Geometry check sheet. Reference: the model listing, model coordinates, mm. Face numbers are marked on the shaded views. A direction names the side the tool comes from. Give positions to 0.01 mm unless a question says otherwise; leave off trailing zeros. Write each loop counter-clockwise with the first axis right and the second up, starting at its lowest first coordinate (ties: lowest second). Pieces come first, ordered by that corner, then holes. Notation, with made-up numbers: (34, 12.25) -> (74, 12.25) arc R26 ccw to (74, 37.25) -> close; hole circle Ø7 at (66, 27.25). An arc over 180 degrees is marked (long way). One line per item, written item: value.
from build123d import *

# Parameters (mm, degrees)
SKETCH1_W           = 21
SKETCH1_H           = 16
SKETCH1_W_2         = 17
SKETCH1_H_2         = 12
BOSS_EXTRUDE1_DEPTH = 2
SKETCH1_6_W         = 21
SKETCH1_6_H         = 16
SKETCH1_6_W_2       = 17
SKETCH1_6_H_2       = 12
BOSS_EXTRUDE2_DEPTH = 7
SKETCH2_W           = 41
SKETCH2_H           = 16
BOSS_EXTRUDE3_DEPTH = 2
SKETCH3_W           = 3.5
SKETCH3_H           = 2
CUT_EXTRUDE1_DEPTH  = 33.954514107
SKETCH4_W           = 3.5
SKETCH4_H           = 8
CUT_EXTRUDE2_DEPTH  = 1
CUT_EXTRUDE3_START  = -7
SKETCH5_W           = 2
SKETCH5_H           = 8
SKETCH5_H_2         = 6
CUT_EXTRUDE3_DEPTH  = 7
CUT_EXTRUDE4_DEPTH  = 2
CUT_EXTRUDE5_DEPTH  = 2
SKETCH9_W           = 4
SKETCH9_H           = 4
BOSS_EXTRUDE4_DEPTH = 7
SKETCH10_R          = 0.5
CUT_EXTRUDE6_DEPTH  = 35.84250278
SKETCH11_W          = 3.5
SKETCH11_H          = 8
CUT_EXTRUDE7_DEPTH  = 1
FILLET1_R           = 2


with BuildPart() as part:
    # Sketch1 → Boss-Extrude1 (new body)
    # profile 1 of 2: a face of its own
    with BuildSketch(Plane(origin=(0, 0, 0), x_dir=(1, 0, 0), z_dir=(0, 1, 0))):
        with Locations((-8.5, 6)):
            Rectangle(SKETCH1_W, SKETCH1_H)
        with Locations((-8.5, 6)):
            Rectangle(SKETCH1_W_2, SKETCH1_H_2, mode=Mode.SUBTRACT)
    # profile 2 of 2: a face of its own
    with BuildSketch(Plane(origin=(0, 0, 0), x_dir=(1, 0, 0), z_dir=(0, 1, 0))):
        with Locations((-8.5, 6)):
            Rectangle(SKETCH1_W_2, SKETCH1_H_2)
    extrude(amount=BOSS_EXTRUDE1_DEPTH)

    # Sketch1<6> → Boss-Extrude2 (add)
    with BuildSketch(Plane(origin=(0, 0, 0), x_dir=(1, 0, 0), z_dir=(0, 1, 0))):
        with Locations((-8.5, 6)):
            Rectangle(SKETCH1_6_W, SKETCH1_6_H)
        with Locations((-8.5, 6)):
            Rectangle(SKETCH1_6_W_2, SKETCH1_6_H_2, mode=Mode.SUBTRACT)
    extrude(amount=BOSS_EXTRUDE2_DEPTH)

    # Sketch2 → Boss-Extrude3 (add)
    with BuildSketch(Plane.XZ):
        with Locations((-8.5, -6)):
            Rectangle(SKETCH2_W, SKETCH2_H)
    extrude(amount=BOSS_EXTRUDE3_DEPTH)

    # Sketch3 → Cut-Extrude1 (cut, through all)
    with BuildSketch(Plane(origin=(0, 0, 0), x_dir=(1, 0, 0), z_dir=(0, 1, 0))):
        with Locations((-24.75, 11)):
            Rectangle(SKETCH3_W, SKETCH3_H)
        with Locations((-24.75, 1)):
            Rectangle(SKETCH3_W, SKETCH3_H)
        with Locations((7.75, 11)):
            Rectangle(SKETCH3_W, SKETCH3_H)
        with Locations((7.75, 1)):
            Rectangle(SKETCH3_W, SKETCH3_H)
    extrude(amount=-CUT_EXTRUDE1_DEPTH, mode=Mode.SUBTRACT)

    # Sketch4 → Cut-Extrude2 (cut)
    with BuildSketch(Plane.XZ.offset(2)):
        with Locations((-24.75, -6)):
            Rectangle(SKETCH4_W, SKETCH4_H)
    extrude(amount=-CUT_EXTRUDE2_DEPTH, mode=Mode.SUBTRACT)

    # Sketch5 → Cut-Extrude3 (cut)
    with BuildSketch(Plane(origin=(0, 7, 0), x_dir=(1, 0, 0), z_dir=(0, 1, 0)).offset(CUT_EXTRUDE3_START)):
        with Locations((-18, 6)):
            Rectangle(SKETCH5_W, SKETCH5_H)
        with Locations((1, 9)):
            Rectangle(SKETCH5_W, SKETCH5_H_2)
    extrude(amount=CUT_EXTRUDE3_DEPTH, mode=Mode.SUBTRACT)

    # Sketch7 → Cut-Extrude4 (cut)
    with BuildSketch(Plane(origin=(0, 2, 0), x_dir=(1, 0, 0), z_dir=(0, 1, 0))):
        Polygon((-17, 2), (-17, 0), (0, 0), (0, 6), (0, 12), (-17, 12), (-17, 10), align=None)
    extrude(amount=-CUT_EXTRUDE4_DEPTH, mode=Mode.SUBTRACT)

    # Sketch8 → Cut-Extrude5 (cut)
    with BuildSketch(Plane(origin=(0, 7, 0), x_dir=(1, 0, 0), z_dir=(0, 1, 0))):
        Polygon((-17, 2), (-19, 2), (-19, -2), (2, -2), (2, 6), (0, 6), (0, 0), (-17, 0), align=None)
        Polygon((-19, 10), (-17, 10), (-17, 12), (2, 12), (2, 14), (-19, 14), align=None)
    extrude(amount=-CUT_EXTRUDE5_DEPTH, mode=Mode.SUBTRACT)

    # Sketch9 → Boss-Extrude4 (add)
    with BuildSketch(Plane(origin=(0, 5, 0), x_dir=(1, 0, 0), z_dir=(0, 1, 0))):
        with Locations((-17, 16)):
            Rectangle(SKETCH9_W, SKETCH9_H)
        with Locations((0, 16)):
            Rectangle(SKETCH9_W, SKETCH9_H)
        with Locations((0, -4)):
            Rectangle(SKETCH9_W, SKETCH9_H)
        with Locations((-17, -4)):
            Rectangle(SKETCH9_W, SKETCH9_H)
    extrude(amount=-BOSS_EXTRUDE4_DEPTH)

    # Sketch10 → Cut-Extrude6 (cut, through all)
    with BuildSketch(Plane(origin=(0, 5, 0), x_dir=(1, 0, 0), z_dir=(0, 1, 0))):
        with Locations(Location((-17, 16, 0), (0, 0, 270))):
            Circle(SKETCH10_R)
        with Locations(Location((0, 16, 0), (0, 0, 270))):
            Circle(SKETCH10_R)
        with Locations(Location((0, -4, 0), (0, 0, 270))):
            Circle(SKETCH10_R)
        with Locations(Location((-17, -4, 0), (0, 0, 270))):
            Circle(SKETCH10_R)
    extrude(amount=-CUT_EXTRUDE6_DEPTH, mode=Mode.SUBTRACT)

    # Sketch11 → Cut-Extrude7 (cut)
    with BuildSketch(Plane.XZ.offset(2)):
        with Locations((7.75, -6)):
            Rectangle(SKETCH11_W, SKETCH11_H)
    extrude(amount=-CUT_EXTRUDE7_DEPTH, mode=Mode.SUBTRACT)

    # Fillet1
    fillet1_edges = [part.edges().sort_by_distance(p)[0] for p in [
        (-29, -1, 2),
        (-29, -1, -14),
        (12, -1, -14),
        (12, -1, 2),
    ]]
    fillet(fillet1_edges, radius=FILLET1_R)


solid = part.part
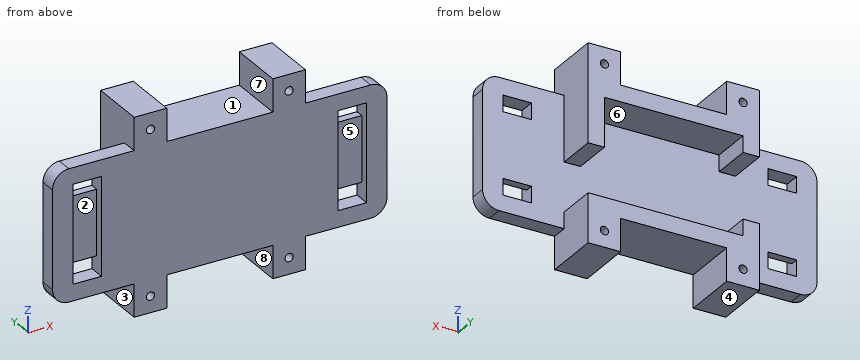
1) Sectioned sample at C-C on z = -16. Record the cut outline in (x, y).
Verdict:
outline: (-19, -2) -> (-17.5, -2) -> (-17.5, 5) -> (-19, 5) -> close; (-16.5, -2) -> (-15, -2) -> (-15, 5) -> (-16.5, 5) -> close; (-2, -2) -> (-0.5, -2) -> (-0.5, 5) -> (-2, 5) -> close; (0.5, -2) -> (2, -2) -> (2, 5) -> (0.5, 5) -> close
2) Sectioned sample at A-A on y = 1.5. Record the cut outline in (x, z).
Verdict:
outline: (-19, -18) -> (-15, -18) -> (-15, -14) -> (-2, -14) -> (-2, -18) -> (2, -18) -> (2, -12) -> (-17, -12) -> (-17, -10) -> (-19, -10) -> close; (-19, -2) -> (-17, -2) -> (-17, 0) -> (0, 0) -> (0, -6) -> (2, -6) -> (2, 6) -> (-2, 6) -> (-2, 2) -> (-15, 2) -> (-15, 6) -> (-19, 6) -> close; hole circle Ø1 at (-17, -16); hole circle Ø1 at (-17, 4); hole circle Ø1 at (0, -16); hole circle Ø1 at (0, 4)
3) Sectioned sample at B-B on z = -5.25. Record the cut outline in (x, y), plus the area to 3 significant figures.
Verdict:
outline: (-29, -2) -> (-26.5, -2) -> (-26.5, -1) -> (-23, -1) -> (-23, -2) -> (6, -2) -> (6, -1) -> (9.5, -1) -> (9.5, -2) -> (12, -2) -> (12, 0) -> (2, 0) -> (2, 5) -> (0, 5) -> (0, 0) -> (-29, 0) -> close
area: 85.0 mm^2
4) Depth check by flat-ended pin: pin 1 Ø3 at (y, z) = (4, -13.5) entering from +X; pin 2 Ø2 at (x, y) = (-10.5, 1.5) entering from +Z; pin 3 Ø0.8 at (x, y) = (-24, -0.5) entering from -Z. Enter the tip coordinate at first touch or a pass-through.
Verdict:
pin 1: x = 2
pin 2: z = 2
pin 3: z = -14
5) Sectioned sample at D-D on x = -14. Record the cut outline in (y, z).
Verdict:
outline: (-2, -14) -> (5, -14) -> (5, -12) -> (0, -12) -> (0, 0) -> (5, 0) -> (5, 2) -> (-2, 2) -> close
6) Mould release check, pull along Z, two halves, no side actions. Record for the marked faces 1, 2, 3 and 4: released by +Z, released by -Z, zero draft, split by the parting line, or undercut.
Verdict:
face 1: released by +Z
face 2: undercut
face 3: zero draft
face 4: released by -Z
7) Scan lines: probe 1 along X at (y, z) = (3, -16); probe 2 along Z at (x, y) = (-9, 1.25); probe 3 along X at (y, z) = (3.75, -1). Record each from-to range of solid material in increasing order.
Verdict:
probe 1: -19 to -17.5, -16.5 to -15, -2 to -0.5, 0.5 to 2
probe 2: -14 to -12, 0 to 2
probe 3: -19 to -17, 0 to 2
8) Tool access check on the marked faces 5, 6, 7 and 8. Record the directions out of +Z, -Z, +X, -X, +Y, -Y that give a thin tool (end or side, any length) a straight path to the whole face; none if there is none.
Verdict:
face 5: -Y
face 6: +Y
face 7: +Z, +Y, -Y
face 8: -Z, +Y, -Y
